Here's how the part is built. I have some questions about the finished solid (model axes, mm). A direction names the side the tool comes from. Give positions to 0.01 mm unless a question says otherwise; leave off trailing zeros. Loops run counter-clockwise (first coordinate to the right, second up) from the corner with the lowest first, then second, coordinate; pieces in that order, holes last. Notation, with made-up numbers: M -12.75,30 L 21.25,30 A25 ccw 21.25,62 Z; hole C -9.75,29 d9. An arc over 180 degrees is marked long. Write item = value, one per line. Start each with the question number.
```python
from build123d import *

# Parameters (mm, degrees)
F0_W     = 8
F0_H     = 1.25
F1_DEPTH = 1.5
F2_DEPTH = 10
F4_DEPTH = 1.25


with BuildPart() as f1:
    # F0 (on Front) → F1 (new body)
    with BuildSketch(Plane.XZ):
        with BuildLine():
            Line((4, 5), (1.5, 5))
            ThreePointArc((1.5, 5), (0, 3.5), (-1.5, 5))
            Line((-1.5, 5), (-4, 5))
            Line((-4, 5), (-4, -3.75))
            Line((-4, -3.75), (4, -3.75))
            Line((4, -3.75), (4, 5))
        make_face()
        with Locations((0, -4.375)):
            Rectangle(F0_W, F0_H)
        with BuildLine():
            ThreePointArc((-1.5, 5), (0, 6.5), (1.5, 5))
            Line((1.5, 5), (4, 5))
            ThreePointArc((4, 5), (0, 9), (-4, 5))
            Line((-4, 5), (-1.5, 5))
        make_face()
    extrude(amount=-F1_DEPTH)

    # F0 (on Front) → F2 (join)
    with BuildSketch(Plane.XZ):
        with Locations((0, -4.375)):
            Rectangle(F0_W, F0_H)
    extrude(amount=F2_DEPTH)

    # F3 (on face) → F4 (cut, through all)
    with BuildSketch(Plane.XY.offset(-3.75)):
        with BuildLine():
            Line((1.414214, -7.414214), (-1.414214, -4.585786))
            ThreePointArc((-1.414214, -4.585786), (-1.414214, -7.414214), (1.414214, -7.414214))
        make_face()
        with BuildLine():
            ThreePointArc((1.414214, -7.414214), (1.847759, -6.765367), (2, -6))
            ThreePointArc((2, -6), (0.765367, -4.152241), (-1.414214, -4.585786))
            Line((-1.414214, -4.585786), (1.414214, -7.414214))
        make_face()
    extrude(amount=-F4_DEPTH, mode=Mode.SUBTRACT)


solid = f1.part
```
Q1. If we section it at B-B, the plane z = 5.25: List the corners of the cut face in (x, y) for me, then the cut area to 3 significant figures.
Q2. On a 3-axis mill with a long thin cutter (end or side, diameter ignored), from which of +Z, -Z, +X, -X, +Y, -Y can I reach the whole of each face in a straight line? I mean faces 4 (the flat face through (0, -10, -4)), 5 (the flat face through (0, 0, 3)). Say none if no direction works.
Q3. Will this pin go through, and if not, where does the flat tip stop? pin 1 (1 mm diameter, centred on x = 0, z = 2.5, fed in from -Y).
Q4. If we section it at A-A, the plane x = 0: List the corners of the cut face in (y, z) for me.
Q5. If we section it at C-C, the plane y = -4.75: List the corners of the cut face in (x, z) for me.
Q6. If I drill on line 1 along Z through (x, y) = (0, 0.65); line 2 along X through (y, z) = (0.75, 5.75); line 3 along Y through (x, z) = (0.5, -2.25), over which ranges is the centre line in solid material (lowest first)?
Q7. We'd pull the mould along Z, two halves only. Please class faces 1 (the cylindrical face through (1.5, 0.74, 5.07)), 2 (the flat face through (-4, 0.5, -1.9)), 3 (the flat face through (-0.1, -3.8, -3.75)): pulls with the +Z half, pulls with the -Z half, needs draft (parallel to the pull), parting line crosses it, or undercut.
Q8. If we section it at D-D, the plane y = 0.75: List the corners of the cut face in (x, z) for me, then the cut area to 3 significant figures.
Resolved:
q1.outline = M -3.99,0 L -1.48,0 L -1.48,1.5 L -3.99,1.5 Z; M 1.48,0 L 3.99,0 L 3.99,1.5 L 1.48,1.5 Z
q1.area = 7.54 mm²
q2.face_4 = +Z, -Z, +X, -X, -Y
q2.face_5 = +Z, +X, -X, -Y
q3.pin_1 = 0
q4.outline = M -10,-5 L -8,-5 L -8,-3.75 L -10,-3.75 Z; M -4,-5 L 1.5,-5 L 1.5,3.5 L 0,3.5 L 0,-3.75 L -4,-3.75 Z; M 0,6.5 L 1.5,6.5 L 1.5,9 L 0,9 Z
q5.outline = M -4,-5 L -1.56,-5 L -1.56,-3.75 L -4,-3.75 Z; M 1.56,-5 L 4,-5 L 4,-3.75 L 1.56,-3.75 Z
q6.line_1 = -5 to 3.5, 6.5 to 9
q6.line_2 = -3.93 to -1.3, 1.3 to 3.93
q6.line_3 = 0 to 1.5
q7.face_1 = undercut
q7.face_2 = needs draft
q7.face_3 = pulls with the +Z half
q8.outline = M -4,-5 L 4,-5 L 4,5 A4 ccw -4,5 Z; hole C 0,5 d3
q8.area = 98.1 mm²
